Source: CAD feature listing. Evaluate the final solid. Frame: model axes, mm. Face numbers are marked on the shaded views. A direction names the side the tool comes from. Round coordinates to 2 decimals unless told otherwise and drop trailing zeros. Write each loop counter-clockwise with the first axis right and the second up, starting at its lowest first coordinate (ties: lowest second). Pieces come first, ordered by that corner, then holes.
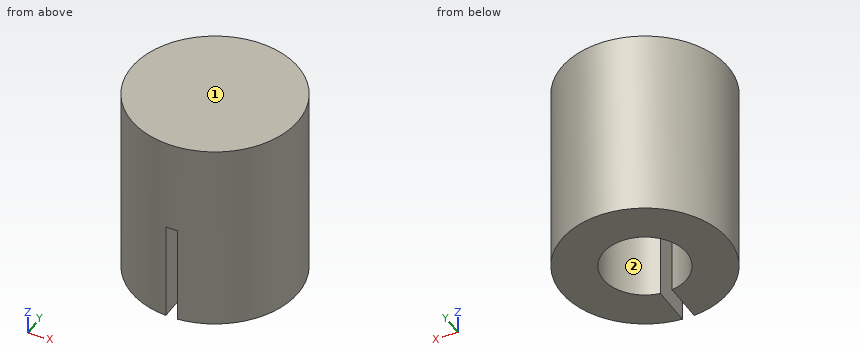
from build123d import *

# Parameters (mm, degrees)
F0_R     = 150.931089
F1_DEPTH = 350
F2_R     = 75.554982
F3_DEPTH = 200
F4_W     = 21.125047
F4_H     = 119.437709
F5_DEPTH = 180


with BuildPart() as f1:
    # F0 (on Top) → F1 (new body)
    with BuildSketch(Plane.XY):
        Circle(F0_R)
    extrude(amount=F1_DEPTH)

    # F2 (on face) → F3 (cut)
    with BuildSketch(Plane(origin=(0, 0, 0), x_dir=(1, 0, 0), z_dir=(0, 0, -1))):
        Circle(F2_R)
    extrude(amount=-F3_DEPTH, mode=Mode.SUBTRACT)

    # F4 (on face) → F5 (cut)
    with BuildSketch(Plane(origin=(0, 0, 0), x_dir=(1, 0, 0), z_dir=(0, 0, -1))):
        with Locations((0.812509, 118.625202)):
            Rectangle(F4_W, F4_H)
    extrude(amount=-F5_DEPTH, mode=Mode.SUBTRACT)


solid = f1.part
1) Section query C-C on z = 149. Return the cut outline in (x, y).
Taken from the geometry:
outline: (-9.75, -150.62) - (-9.75, -74.92) arc R75.55 cw (long way) to (11.38, -74.69) - (11.38, -150.5) arc R150.93 ccw (long way) to start
2) Reachability of the marked faces 1 and 2 from +Z, -Z, +X, -X, +Y, -Y: full face, straight path, thin tool, end or side. Return the list, or none.
Taken from the geometry:
face 1: +Z, +X, -X, +Y, -Y
face 2: -Z
3) Material intervals for line 1 (X direction, y = 0, z = 81); line 2 (Z direction, x = -38, y = -64); line 3 (X direction, y = -35, z = 64), sorted ascending.
Taken from the geometry:
line 1: x = -150.93 to -75.55, 75.55 to 150.93
line 2: z = 200 to 350
line 3: x = -146.82 to -66.96, 66.96 to 146.82
4) Contact query for flat-ended pins moving along their axis: P1, Ø3, axis at y = -93, z = 230.5, coming from the -X side; P2, Ø1.5, axis at x = -8.5, z = 300, coming from the -Y side; P3, Ø3, axis at x = 6, z = 169, coming from the -Y side. Output: stop coordinate, or through.
Taken from the geometry:
P1: stops at x = -120.03
P2: stops at y = -150.73
P3: stops at y = 75.18
5) Section query A-A on y = 0. Return the cut outline in (x, z), then the cut area to 3 significant figures.
Taken from the geometry:
outline: (-150.93, 0) - (-75.55, 0) - (-75.55, 200) - (75.55, 200) - (75.55, 0) - (150.93, 0) - (150.93, 350) - (-150.93, 350) - close
area: 75,400 mm2
6) Section query D-D on z = 195.5. Return the cut outline in (x, y), then the cut area to 3 significant figures.
Taken from the geometry:
outline: circle Ø301.86 at (0, 0); hole circle Ø151.11 at (0, 0)
area: 53,600 mm2
7) Section query B-B on x = 0. Return the cut outline in (y, z).
Taken from the geometry:
outline: (-150.93, 180) - (-75.55, 180) - (-75.55, 200) - (75.55, 200) - (75.55, 0) - (150.93, 0) - (150.93, 350) - (-150.93, 350) - close
